Geometry: final body of the model. Coordinates: model frame, mm. A direction names the side the tool comes from. Give positions to 0.01 mm unless a question says otherwise; leave off trailing zeros. Order: outer loops, then holes, each group sorted by start corner. A loop starts at its lowest first (then second) coordinate and runs counter-clockwise, first axis right, second up. Notation, with made-up numbers: (17, 62.25) - (26, 62.25) arc R17 cw to (26, 70.25) - close; hole circle Ø8 at (-33, -9). An arc over 180 degrees is marked (long way). Put each result on its own line as item: value. Start each with the question number.
1. Section C-C on z = 208.5. Return the cut outline in (x, y), plus the area to 3 significant figures.
2. Section B-B on x = 4.5. Return the cut outline in (y, z), plus the area to 3 significant figures.
3. First-contact query: P1, Ø3, axis at x = 3.5, z = -464.5, coming from the +Y side; P2, Ø3, axis at x = 3.5, y = 107.5, coming from the -Z side; P3, Ø8, axis at y = 40.5, z = 319, coming from the -X side. Flat tips, straight axial feed; report the tip coordinate or a pass-through.
4. Ray query, line 1 along Y through (x, z) = (3, 146); line 2 along Z through (x, y) = (0.75, 90); line 3 along Y through (x, z) = (3.25, -158). Return the intervals inside material, ascending. Write a range as from..to.
5. Mould query, pull axis Z, two halves, no side actions, for faces 3 (the cylindrical face through (3.131, 45.294, 308.529)), 4 (the flat face through (6.35, -32, 7)). Classes: pulls with the +Z half, pulls with the -Z half, needs draft (parallel to the pull), parting line crosses it, or undercut.
6. Set-up query: faces 1 (the cylindrical face through (3.131, 47.071, -234.106)), 2 (the flat face through (0, -30, 7)). Return all of +Z, -Z, +X, -X, +Y, -Y with unobstructed straight access to the full face (end or side cutting, diameter ignored); none if empty.
7. Section D-D on y = 106. Return the cut outline in (x, z).
8. Section A-A on y = 68. Return the cut outline in (x, z), plus the area to 3 significant figures.
from build123d import *

# Parameters (mm, degrees)
F1_DEPTH = 6.35
F2_SIZE  = 4.7625


with BuildPart() as f1:
    # F0 (on Right) → F1 (new body)
    with BuildSketch(Plane.YZ):
        with BuildLine():
            Line((127, 476.25), (-127, 476.25))
            Line((-127, 476.25), (-127, -476.25))
            Line((-127, -476.25), (88.9, -476.25))
            Line((88.9, -476.25), (88.9, -438.15))
            Line((88.9, -438.15), (127, -438.15))
            Line((127, -438.15), (127, -266.7))
            ThreePointArc((127, -266.7), (46.177695, -233.222305), (12.7, -152.4))
            Line((12.7, -152.4), (12.7, 228.6))
            ThreePointArc((12.7, 228.6), (46.177695, 309.422305), (127, 342.9))
            Line((127, 342.9), (127, 476.25))
        make_face()
    extrude(amount=F1_DEPTH)

    # F2
    f2_edges = [f1.edges().sort_by_distance(p)[0] for p in [
        (6.35, 127, 409.575),
        (6.35, 127, -352.425),
    ]]
    chamfer(f2_edges, length=F2_SIZE)


solid = f1.part
Resolved:
1. outline: (0, -127) - (6.35, -127) - (6.35, 12.7) - (0, 12.7) - close
1. area: 887 mm^2
2. outline: (-127, -476.25) - (88.9, -476.25) - (88.9, -438.15) - (124.09, -438.15) - (124.09, -266.66) arc R114.3 cw to (12.7, -152.4) - (12.7, 228.6) arc R114.3 cw to (124.09, 342.86) - (124.09, 476.25) - (-127, 476.25) - close
2. area: 176,000 mm^2
3. P1: y = 88.9
3. P2: z = -438.15
3. P3: x = 0
4. line 1: -127..12.7
4. line 2: -438.15..-260.55, 336.75..476.25
4. line 3: -127..12.84
5. face 3: undercut
5. face 4: needs draft
6. face 1: +X, -X, +Y
6. face 2: +Z, -Z, -X, +Y, -Y
7. outline: (0, -438.15) - (6.35, -438.15) - (6.35, -264.75) - (0, -264.75) - close; (0, 340.95) - (6.35, 340.95) - (6.35, 476.25) - (0, 476.25) - close
8. outline: (0, -476.25) - (6.35, -476.25) - (6.35, -250.3) - (0, -250.3) - close; (0, 326.5) - (6.35, 326.5) - (6.35, 476.25) - (0, 476.25) - close
8. area: 2,390 mm^2
